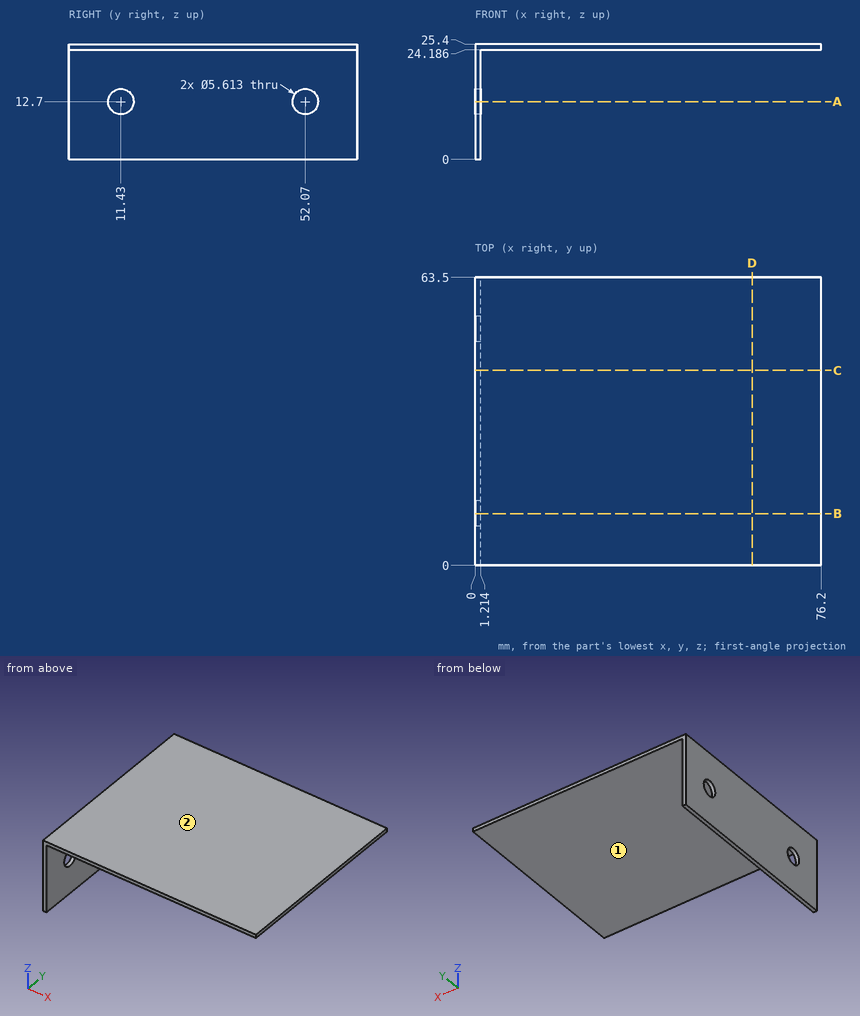
The drawing under review shows one solid part. Ordinate dimensions are in mm from its lowest x, y, z. A direction names the side the tool comes from. Coordinates: 2 decimals unless noted, no trailing zeros. Loops run counter-clockwise (first coordinate to the right, second up) from the corner with the lowest first, then second, coordinate; pieces in that order, holes last. Notation, with made-up numbers: (89.5, -34) - (126.5, -34) arc R30 cw to (126.5, -11) - close; hole circle Ø5 at (-14.5, 25.25). An arc over 180 degrees is marked (long way). Return JSON: item names as keys, results as strings.
Item 1: Take a section at C-C (y = 43). Give the boundary of the cut face in (x, z).
Determined:
{"outline": "(0, 0) - (1.21, 0) - (1.21, 24.19) - (76.2, 24.19) - (76.2, 25.4) - (0, 25.4) - close"}
Item 2: Take a section at D-D (x = 61). Give the boundary of the cut face in (y, z).
Determined:
{"outline": "(0, 24.19) - (63.5, 24.19) - (63.5, 25.4) - (0, 25.4) - close"}
Item 3: Insertion check: pin 1 (1.5 mm diameter, centred on y = 8, z = 15, fed in from -X); pin 2 (4.5 mm diameter, centred on y = 11.43, z = 12.7, fed in from +X); pin 3 (1.5 mm diameter, centred on x = 21.5, y = 17.5, fed in from -Z); pin 4 (2 mm diameter, centred on y = 47.5, z = 7, fed in from +X). Each pin has a flat end and moves straight along its axis. Give the tip position at first contact, or say it passes through.
Determined:
{"pin 1": "stops at x = 0", "pin 2": "passes through", "pin 3": "stops at z = 24.19", "pin 4": "stops at x = 1.21"}
Item 4: Take a section at B-B (y = 11.43). Give the boundary of the cut face in (x, z), then the cut area to 3 significant figures.
Determined:
{"outline": "(0, 0) - (1.21, 0) - (1.21, 9.89) - (0, 9.89) - close; (0, 15.51) - (1.21, 15.51) - (1.21, 24.19) - (76.2, 24.19) - (76.2, 25.4) - (0, 25.4) - close", "area": "115 mm2"}
Item 5: For the marked faces 1 and 2, list the 3-axis set-ups (+Z, -Z, +X, -X, +Y, -Y) from which the entire face can be reached by the end or side of a thin tool; tool diameter is ignored.
Determined:
{"face 1": "-Z, +X, +Y, -Y", "face 2": "+Z, +X, -X, +Y, -Y"}
Item 6: Take a section at A-A (z = 12.7). Give the boundary of the cut face in (x, y).
Determined:
{"outline": "(0, 0) - (1.21, 0) - (1.21, 8.62) - (0, 8.62) - close; (0, 14.24) - (1.21, 14.24) - (1.21, 49.26) - (0, 49.26) - close; (0, 54.88) - (1.21, 54.88) - (1.21, 63.5) - (0, 63.5) - close"}
Item 7: For line 1 (Y direction, x = 0.95, z = 12.7); line 2 (X direction, y = 40, z = 4.75); line 3 (Z direction, x = 18, y = 26), list the stretches that pass through material, from the lowest coordinate up.
Determined:
{"line 1": "y = 0 to 8.62, 14.24 to 49.26, 54.88 to 63.5", "line 2": "x = 0 to 1.21", "line 3": "z = 24.19 to 25.4"}
